Print and shaded views of the part. All mm, measured from the part's lowest x, y and z. Give positions to 0.01 mm unless a question says otherwise; leave off trailing zeros. Loops run counter-clockwise (first coordinate to the right, second up) from the corner with the lowest first, then second, coordinate; pieces in that order, holes last. Notation, with made-up numbers: M 77,44 L 110,44 A31 cw 110,77 Z; hole C 79,86.25 d5. An arc over 180 degrees is marked long. Put each result on its own line as item: value. Start each with the question number.
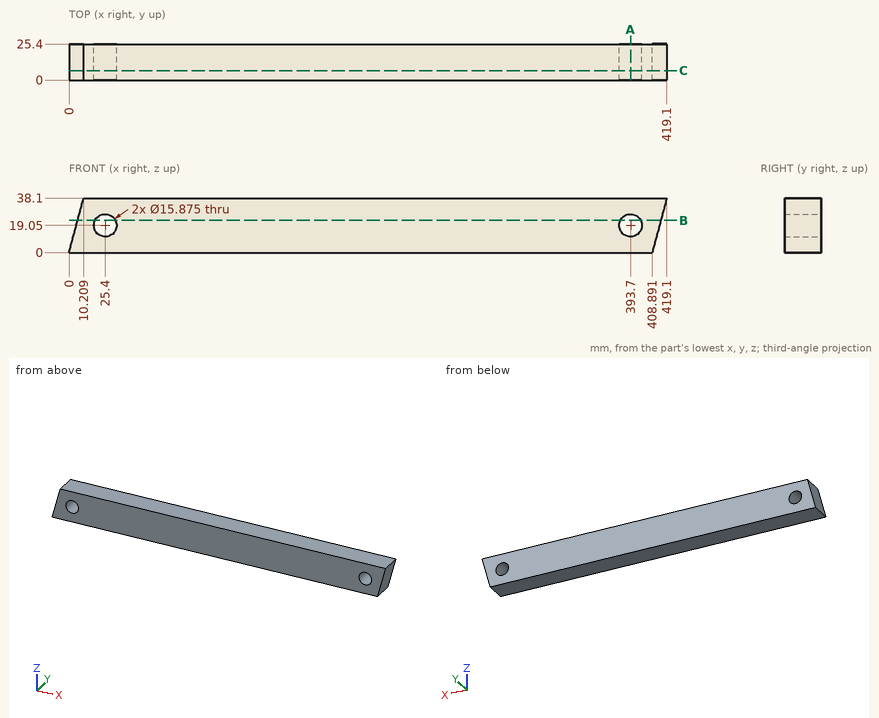
1) Wall check: L1, parallel to Z at x = 25.4, y = 19.25; L2, parallel to X at y = 6.5, z = 26 (1 decimal); L3, parallel to Z at x = 28, y = 20.75. Give the ranges that are in metal, low to high.
2) Band-saw the part on C-C on y = 6.75. State how many separate pieces and enclosed holes the cut face has, then the cut area to 3 significant figures.
3) Pin check, flat tips, straight feed: pin 1 Ø5 at (y, z) = (11.5, 16) entering from +X; pin 2 Ø1.5 at (y, z) = (20, 16) entering from -X; pin 3 Ø2 at (y, z) = (4.5, 22.5) entering from -X. Stop position of each tip, or through.
4) Band-saw the part on A-A on x = 393.7. Give the cut face in (y, z).
5) Band-saw the part on B-B on z = 22.5. Give the cut face in (x, y).
Evaluation:
1. L1: 0 to 11.11, 26.99 to 38.1
1. L2: 7 to 21.6, 29.2 to 389.9, 397.5 to 415.9
1. L3: 0 to 11.55, 26.55 to 38.1
2. separate pieces: 1
2. enclosed holes: 2
2. area: 15,200 mm2
3. pin 1: x = 413.85
3. pin 2: x = 4.09
3. pin 3: x = 5.76
4. outline: M 0,0 L 25.4,0 L 25.4,11.11 L 0,11.11 Z; M 0,26.99 L 25.4,26.99 L 25.4,38.1 L 0,38.1 Z
5. outline: M 6.03,0 L 18.25,0 L 18.25,25.4 L 6.03,25.4 Z; M 32.55,0 L 386.55,0 L 386.55,25.4 L 32.55,25.4 Z; M 400.85,0 L 414.92,0 L 414.92,25.4 L 400.85,25.4 Z
